Verification items for the finished model (mm, model axes). A direction names the side the tool comes from. Coordinates: 2 decimals unless noted, no trailing zeros. Write each loop counter-clockwise with the first axis right and the second up, starting at its lowest first coordinate (ties: lowest second). Pieces come first, ordered by that corner, then holes. Notation, with made-up numbers: M -10,44.25 L 22,44.25 A21 cw 22,60.25 Z; hole C 80,56 d3. An arc over 180 degrees is marked long. Answer in a Markdown table with one row per item.
from build123d import *

# Parameters (mm, degrees)
SKETCH2_W           = 177.8
SKETCH2_H           = 152.4
BOSS_EXTRUDE1_DEPTH = 76.2
SKETCH10_W          = 76.2
SKETCH10_H          = 50.8
CUT_EXTRUDE2_DEPTH  = 193.18587357
SKETCH12_W          = 76.2
SKETCH12_H          = 25.4
CUT_EXTRUDE3_DEPTH  = 156.02325632
CUT_EXTRUDE4_DEPTH  = 208.907960406


with BuildPart() as part:
    # Sketch2 → Boss-Extrude1 (new, symmetric)
    with BuildSketch(Plane.XY):
        Rectangle(SKETCH2_W, SKETCH2_H)
    extrude(amount=BOSS_EXTRUDE1_DEPTH, both=True)

    # Sketch10 → Cut-Extrude2 (cut, through all)
    with BuildSketch(Plane.XY.offset(76.2)):
        with Locations((0, 50.8)):
            Rectangle(SKETCH10_W, SKETCH10_H)
    extrude(amount=-CUT_EXTRUDE2_DEPTH, mode=Mode.SUBTRACT)

    # Sketch12 → Cut-Extrude3 (cut, through all)
    with BuildSketch(Plane(origin=(0, 25.4, 0), x_dir=(1, 0, 0), z_dir=(0, 1, 0))):
        with Locations((0, -63.5)):
            Rectangle(SKETCH12_W, SKETCH12_H)
        with Locations((0, 63.5)):
            Rectangle(SKETCH12_W, SKETCH12_H)
    extrude(amount=-CUT_EXTRUDE3_DEPTH, mode=Mode.SUBTRACT)

    # Sketch13 → Cut-Extrude4 (cut, through all)
    with BuildSketch(Plane(origin=(88.9, 0, 0), x_dir=(0, 0, -1), z_dir=(1, 0, 0))):
        Polygon((76.2, 76.2), (0, 76.2), (76.2, 0), align=None)
        Polygon((-76.2, 76.2), (-76.2, 0), (0, 76.2), align=None)
    extrude(amount=-CUT_EXTRUDE4_DEPTH, mode=Mode.SUBTRACT)


solid = part.part
1) Release check for a two-part mould opening along X. For faces 1 (the face through (-63.1, 37.6, 38.6)), 2 (the face through (88.9, -18, 1)), 3 (the face through (-1, -25, 50.8)) record: +X half, -X half, draft (parallel to the pull), parting line (faces both ways), or undercut.
Response values:
| item | result |
|---|---|
| face 1 | draft |
| face 2 | +X half |
| face 3 | undercut |
2) Sectioned sample at D-D (x = 60.5). Record the cut outline in (y, z), then the cut area to 3 significant figures.
Response values:
| item | result |
|---|---|
| outline | M -76.2,-76.2 L 0,-76.2 L 76.2,0 L 0,76.2 L -76.2,76.2 Z |
| area | 17,400 mm² |
3) Tool access check on faces 4 (the face through (-38.1, 46, 1)), 5 (the face through (-38.1, -36, -63)), 6 (the face through (-38.1, -36, 64)). Record the directions out of +Z, -Z, +X, -X, +Y, -Y that give a thin tool (end or side, any length) a straight path to the whole face; none if there is none.
Response values:
| item | result |
|---|---|
| face 4 | +Z, -Z, +Y |
| face 5 | -Z, +Y, -Y |
| face 6 | +Z, +Y, -Y |
4) Sectioned sample at B-B (z = -42). Record the cut outline in (x, y).
Response values:
| item | result |
|---|---|
| outline | M -88.9,-76.2 L 88.9,-76.2 L 88.9,34.2 L 38.1,34.2 L 38.1,25.4 L -38.1,25.4 L -38.1,34.2 L -88.9,34.2 Z |
5) Depth check by flat-ended pin: pin 1 (1.5 mm diameter, centred on x = -11.5, z = -41.5, fed in from +Y); pin 2 (5 mm diameter, centred on x = -68.5, z = 29, fed in from +Y); pin 3 (5 mm diameter, centred on x = -10.5, y = -26, fed in from +Z). Enter the tip coordinate at first touch or a pass-through.
Response values:
| item | result |
|---|---|
| pin 1 | stops at y = 25.4 |
| pin 2 | stops at y = 49.7 |
| pin 3 | stops at z = 50.8 |
6) Sectioned sample at C-C (y = 19). Record the cut outline in (x, z), then the cut area to 3 significant figures.
Response values:
| item | result |
|---|---|
| outline | M -88.9,-57.2 L -38.1,-57.2 L -38.1,-50.8 L 38.1,-50.8 L 38.1,-57.2 L 88.9,-57.2 L 88.9,57.2 L 38.1,57.2 L 38.1,50.8 L -38.1,50.8 L -38.1,57.2 L -88.9,57.2 Z |
| area | 19,400 mm² |
7) Thickness scan on L1, parallel to X at y = 34, z = -25; L2, parallel to Y at x = -29, z = 50; L3, parallel to Z at x = -15.5, y = -40.5. Record the ranges inside material, lowest first. Write a range as [from, to].
Response values:
| item | result |
|---|---|
| L1 | x = [-88.9, -38.1], [38.1, 88.9] |
| L2 | y = [-76.2, 25.4] |
| L3 | z = [-50.8, 50.8] |
8) Sectioned sample at A-A (y = 54). Record the cut outline in (x, z).
Response values:
| item | result |
|---|---|
| outline | M -88.9,-22.2 L -38.1,-22.2 L -38.1,22.2 L -88.9,22.2 Z; M 38.1,-22.2 L 88.9,-22.2 L 88.9,22.2 L 38.1,22.2 Z |
